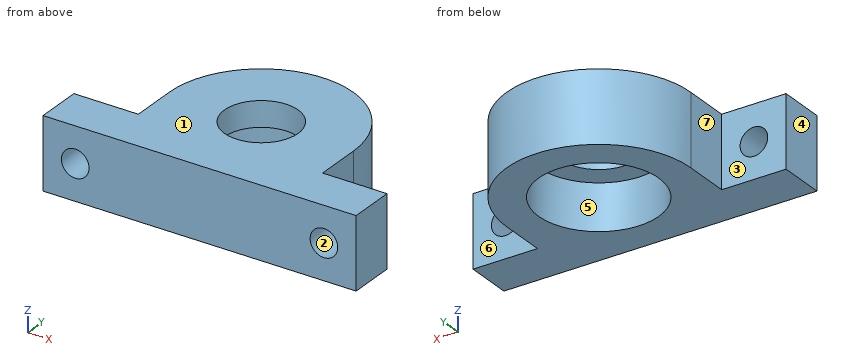
```python
from build123d import *

# Parameters (mm, degrees)
SKETCH1_R           = 13.05
BOSS_EXTRUDE1_DEPTH = 10
SKETCH2_R           = 8
BOSS_EXTRUDE2_DEPTH = 5.5
SKETCH3_R           = 3
CUT_EXTRUDE1_DEPTH  = 11


with BuildPart() as part:
    # Sketch1 → Boss-Extrude1 (new body)
    with BuildSketch(Plane.XY):
        with BuildLine():
            Line((-34, 0), (34, 0))
            Line((34, 0), (34, 10))
            Line((34, 10), (20, 10))
            Line((20, 10), (20, 20))
            ThreePointArc((20, 20), (0, 40), (-20, 20))
            Line((-20, 20), (-20, 10))
            Line((-20, 10), (-34, 10))
            Line((-34, 10), (-34, 0))
        make_face()
        with Locations((0, 20)):
            Circle(SKETCH1_R, mode=Mode.SUBTRACT)
    extrude(amount=BOSS_EXTRUDE1_DEPTH)

    # Sketch2 → Boss-Extrude2 (add)
    with BuildSketch(Plane.XY.offset(10)):
        with BuildLine():
            Line((34, 0), (34, 10))
            Line((34, 10), (20, 10))
            Line((20, 10), (20, 20))
            ThreePointArc((20, 20), (0, 40), (-20, 20))
            Line((-20, 20), (-20, 10))
            Line((-20, 10), (-34, 10))
            Line((-34, 10), (-34, 0))
            Line((-34, 0), (34, 0))
        make_face()
        with Locations((0, 20)):
            Circle(SKETCH2_R, mode=Mode.SUBTRACT)
    extrude(amount=BOSS_EXTRUDE2_DEPTH)

    # Sketch3 → Cut-Extrude1 (cut, through all)
    with BuildSketch(Plane(origin=(0, 10, 0), x_dir=(1, 0, 0), z_dir=(0, 1, 0))):
        with Locations((27, -7.75)):
            Circle(SKETCH3_R)
        with Locations((-27, -7.75)):
            Circle(SKETCH3_R)
    extrude(amount=-CUT_EXTRUDE1_DEPTH, mode=Mode.SUBTRACT)


solid = part.part
```
Design review of the part built by this model. Coordinates are the model's own, in mm. Face numbers are marked on the shaded views. A direction names the side the tool comes from. Round coordinates to 2 decimals unless told otherwise and drop trailing zeros. Write each loop counter-clockwise with the first axis right and the second up, starting at its lowest first coordinate (ties: lowest second). Pieces come first, ordered by that corner, then holes. Notation, with made-up numbers: (85.25, 68) -> (104.25, 68) arc R13 cw to (104.25, 74) -> close; hole circle Ø11 at (41, 28.25). An arc over 180 degrees is marked (long way). Write item = value, one per line. Start each with the question number.
1) Mouldability with a two-part tool opening along Z and no side actions: class the marked faces 1, 2 and 3 as +Z half, -Z half, draft (parallel to the pull), parting line (faces both ways), or undercut.
2) Take a section at D-D, the plane y = 17.5. State the section outline as (x, z) points.
3) Wall thickness on probe 1 along Y at (x, z) = (0, 13.8); probe 2 along X at (y, z) = (16, 3.5); probe 3 along Y at (x, z) = (-7, 13.25) (3 decimals): over which ranges is each line inside the solid? List them lowest first. Write a range as from..to.
4) Take a section at A-A, the plane z = 7.75. State the section outline as (x, y) points, plus the area to 3 significant figures.
5) Take a section at B-B, the plane x = 27. State the section outline as (y, z) points.
6) Take a section at C-C, the plane z = 12. State the section outline as (x, y) points.
7) Tool access review of the marked faces 4, 5, 6 and 7: name each direction out of +Z, -Z, +X, -X, +Y, -Y from which nothing blocks a thin tool from reaching the whole face with its end or side.
8) Clearance check with flat-ended pins moving along their axes: pin 1 (8 mm diameter, centred on y = 13.5, z = 13, fed in from +X); pin 2 (2 mm diameter, centred on y = 15, z = 11.5, fed in from -X); pin 3 (1 mm diameter, centred on x = 2, z = 5, fed in from +Y); pin 4 (5 mm diameter, centred on y = 17, z = 8.5, fed in from +X). State where each tip first meets the part, or that it passes through.
Results list:
q1.face_1 = +Z half
q1.face_2 = undercut
q1.face_3 = draft
q2.outline = (-20, 0) -> (-12.81, 0) -> (-12.81, 10) -> (-7.6, 10) -> (-7.6, 15.5) -> (-20, 15.5) -> close; (7.6, 10) -> (12.81, 10) -> (12.81, 0) -> (20, 0) -> (20, 15.5) -> (7.6, 15.5) -> close
q3.probe_1 = 0..12, 28..40
q3.probe_2 = -20..-12.42, 12.42..20
q3.probe_3 = 0..16.127, 23.873..38.735
q4.outline = (-34, 0) -> (-30, 0) -> (-30, 10) -> (-34, 10) -> close; (-24, 0) -> (24, 0) -> (24, 10) -> (20, 10) -> (20, 20) arc R20 ccw to (-20, 20) -> (-20, 10) -> (-24, 10) -> close; (30, 0) -> (34, 0) -> (34, 10) -> (30, 10) -> close; hole circle Ø26.1 at (0, 20)
q4.area = 1,050 mm²
q5.outline = (0, 0) -> (10, 0) -> (10, 4.75) -> (0, 4.75) -> close; (0, 10.75) -> (10, 10.75) -> (10, 15.5) -> (0, 15.5) -> close
q6.outline = (-34, 0) -> (34, 0) -> (34, 10) -> (20, 10) -> (20, 20) arc R20 ccw to (-20, 20) -> (-20, 10) -> (-34, 10) -> close; hole circle Ø16 at (0, 20)
q7.face_4 = +Z, -Z, -X, +Y, -Y
q7.face_5 = -Z
q7.face_6 = +Z, -Z, +X, +Y
q7.face_7 = +Z, -Z, -X, +Y
q8.pin_1 = 34
q8.pin_2 = -20
q8.pin_3 = 39.94
q8.pin_4 = 20
